Source: CAD feature listing. Evaluate the final solid. Frame: model axes, mm. Round coordinates to 2 decimals unless told otherwise and drop trailing zeros. Write each loop counter-clockwise with the first axis right and the second up, starting at its lowest first coordinate (ties: lowest second). Pieces come first, ordered by that corner, then holes.
Autodesk Inventor part; units mm, degrees
ref_plane "YZ Plane" through (0, 0, 0) normal (1, 0, 0) x (0, 1, 0)
ref_plane "XZ Plane" through (0, 0, 0) normal (0, 1, 0) x (-1, 0, 0)
ref_plane "XY Plane" through (0, 0, 0) normal (0, 0, 1) x (1, 0, 0)
sketch "Sketch1" plane through (0, 0, 0) normal (0, 1, 0) x (-1, 0, 0)
  circle A0 centre (0, 0) radius 36.14
  dimension "d0" = 72.28
extrude "Extrusion1" add sketch "Sketch1" along normal blind 100 draft 4
shell "Shell1" thickness 0.38 removed faces 2 at (-7.9764, 0, 7.1147) at (-8.1176, 100, 9.5927)
properties part number "E"
1) Section query B-B on x = 0. Return the cut outline in (y, z).
Taken from the geometry:
outline: (0, -36.14) - (100, -43.13) - (100, -42.75) - (0, -35.76) - close; (0, 35.76) - (100, 42.75) - (100, 43.13) - (0, 36.14) - close
2) Section query D-D on y = 42.5. Return the cut outline in (x, z).
Taken from the geometry:
outline: circle Ø78.22 at (0, 0); hole circle Ø77.46 at (0, 0)
3) Section query A-A on z = 0. Return the cut outline in (x, y), then the cut area to 3 significant figures.
Taken from the geometry:
outline: (-43.13, 100) - (-36.14, 0) - (-35.76, 0) - (-42.75, 100) - close; (35.76, 0) - (36.14, 0) - (43.13, 100) - (42.75, 100) - close
area: 76.2 mm2
4) Pull-direction query (X, two-part tool) for faces 1 (the face through (8.52, 50.7, -38.37)), 2 (the face through (-9, 100, 42)), 3 (the face through (-37.853, 50.7, 11.92)); classes: released by +X, released by -X, zero draft, split by the parting line, or undercut.
Taken from the geometry:
face 1: undercut
face 2: zero draft
face 3: split by the parting line
5) Section query C-C on y = 54. Return the cut outline in (x, z).
Taken from the geometry:
outline: circle Ø79.83 at (0, 0); hole circle Ø79.07 at (0, 0)
6) Contact query for flat-ended pins moving along their axis: P1, Ø1.5, axis at y = 78.5, z = -4.5, coming from the +X side; P2, Ø10, axis at y = 63, z = 23.5, coming from the -X side; P3, Ø2, axis at y = 86, z = -30, coming from the -X side. Output: stop coordinate, or through.
Taken from the geometry:
P1: stops at x = 41.48
P2: stops at x = -36.11
P3: stops at x = -30.6
7) Material intervals for line 1 (X direction, y = 15, z = 10.5); line 2 (Z direction, x = -16, y = 32); line 3 (X direction, y = 95, z = 15), sorted ascending.
Taken from the geometry:
line 1: x = -35.68 to -35.28, 35.28 to 35.68
line 2: z = -34.88 to -34.46, 34.46 to 34.88
line 3: x = -40.07 to -39.66, 39.66 to 40.07
